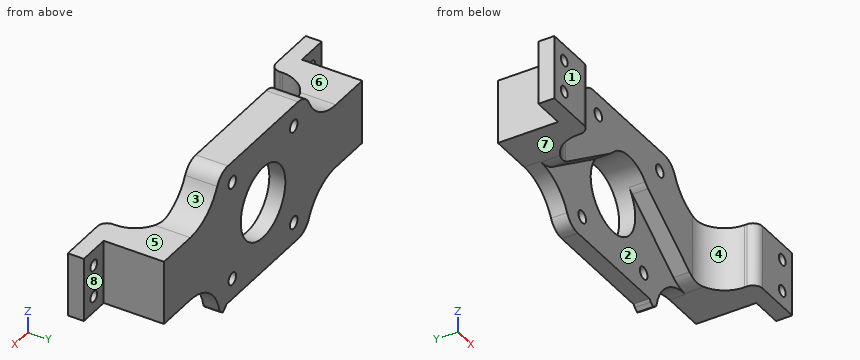
```python
from build123d import *

# Parameters (mm, degrees)
AUFSATZ_LINEAR_AUSTRAGEN1_DEPTH      = 10
SKIZZE6_R                            = 1.9
SKIZZE6_R_2                          = 11.25
SCHNITT_LINEAR_AUSTRAGEN4_DEPTH      = 67.632124385
SKIZZE7_W                            = 20.880821379
SKIZZE7_H                            = 5
SCHNITT_LINEAR_AUSTRAGEN5_DEPTH      = 87.970339772
VERRUNDUNG3_R                        = 15
SCHNITT_LINEAR_AUSTRAGEN6_DEPTH      = 69.73136111
SCHNITT_LINEAR_AUSTRAGEN6_DEPTH_BACK = 69.73136111
SKIZZE8_W                            = 10
SKIZZE8_H                            = 10
AUFSATZ_LINEAR_AUSTRAGEN4_DEPTH      = 20
VERRUNDUNG7_R                        = 10
VERRUNDUNG8_R                        = 3
SKIZZE16_R                           = 1.7
SCHNITT_LINEAR_AUSTRAGEN8_DEPTH      = 10
AUFSATZ_LINEAR_AUSTRAGEN6_DEPTH      = 5
VERRUNDUNG9_R                        = 0.5
FASE1_START                          = -13.795598923
FASE1_DEPTH                          = 18.795598923
VERRUNDUNG10_R                       = 10
VERRUNDUNG11_R                       = 6


with BuildPart() as part:
    # Skizze1 → Aufsatz-Linear austragen1 (new body)
    with BuildSketch(Plane(origin=(0, 0, 0), x_dir=(1, 0, 0), z_dir=(0, 1, 0))):
        Polygon((-60, -4.8), (-22, -4.8), (-22, -16.8), (22, -16.8), (22, -4.8), (60, -4.8), (60, 15.2), (22, 15.2), (22, 27.2), (0, 27.2), (-22, 27.2), (-22, 15.2), (-60, 15.2), align=None)
    extrude(amount=AUFSATZ_LINEAR_AUSTRAGEN1_DEPTH)

    # Skizze6 → Schnitt-Linear austragen4 (cut, through all)
    with BuildSketch(Plane(origin=(0, 10, 0), x_dir=(1, 0, 0), z_dir=(0, 1, 0))):
        with Locations(Location((15.5, 20.7, 0), (0, 0, 270))):
            Circle(SKIZZE6_R)
        with Locations(Location((15.5, -10.3, 0), (0, 0, 270))):
            Circle(SKIZZE6_R)
        with Locations(Location((-15.5, -10.3, 0), (0, 0, 270))):
            Circle(SKIZZE6_R)
        with Locations(Location((-15.5, 20.7, 0), (0, 0, 270))):
            Circle(SKIZZE6_R)
        with Locations(Location((0, 5.2, 0), (0, 0, 270))):
            Circle(SKIZZE6_R_2)
    extrude(amount=-SCHNITT_LINEAR_AUSTRAGEN4_DEPTH, mode=Mode.SUBTRACT)

    # Skizze7 → Schnitt-Linear austragen5 (cut, through all)
    with BuildSketch(Plane.ZY.offset(22)):
        with Locations((-25.64041069, 2.5)):
            Rectangle(SKIZZE7_W, SKIZZE7_H)
    extrude(amount=-SCHNITT_LINEAR_AUSTRAGEN5_DEPTH, mode=Mode.SUBTRACT)

    # Verrundung3
    # the kernel refuses this fillet: 15 mm, written as the material it adds along each edge
    with BuildSketch(Plane(origin=(-22, 5, -15.2), x_dir=(0, 0, -1), z_dir=(0, 1, 0))) as verrundung3_piece_1:
        with BuildLine():
            CenterArc((15, 14.696938457), VERRUNDUNG3_R, 180, 78.463040967)
            Line((0, 14.696938457), (-0.3, 14.696938457))
            Line((-0.3, 14.696938457), (-0.3, 0))
            Line((-0.3, 0), (0, -0.3))
            ThreePointArc((0, -0.3), (6, -0.3), (11.94, -0.293938769))
            Line((11.94, -0.293938769), (12, 0))
        make_face()
    extrude(amount=5)
    with BuildSketch(Plane(origin=(-22, 0, 4.8), x_dir=(-1, 0, 0), z_dir=(0, 1, 0))) as verrundung3_piece_2:
        with BuildLine():
            CenterArc((14.696938457, 15), VERRUNDUNG3_R, 191.536959033, 78.463040967)
            Line((0, 12), (-0.293938769, 11.94))
            ThreePointArc((-0.293938769, 11.94), (-0.3, 6), (-0.3, 0))
            Line((-0.3, 0), (0, -0.3))
            Line((0, -0.3), (14.696938457, -0.3))
            Line((14.696938457, -0.3), (14.696938457, 0))
        make_face()
    extrude(amount=10)
    with BuildSketch(Plane(origin=(22, 0, 4.8), x_dir=(1, 0, 0), z_dir=(0, 1, 0))) as verrundung3_piece_3:
        with BuildLine():
            CenterArc((14.696938457, -15), VERRUNDUNG3_R, 90, 78.463040967)
            Line((0, -12), (-0.293938769, -11.94))
            ThreePointArc((-0.293938769, -11.94), (-0.3, -6), (-0.3, 0))
            Line((-0.3, 0), (0, 0.3))
            Line((0, 0.3), (14.696938457, 0.3))
            Line((14.696938457, 0.3), (14.696938457, 0))
        make_face()
    extrude(amount=10)
    with BuildSketch(Plane(origin=(22, 5, -15.2), x_dir=(1, 0, 0), z_dir=(0, 1, 0))) as verrundung3_piece_4:
        with BuildLine():
            CenterArc((14.696938457, 15), VERRUNDUNG3_R, 191.536959033, 78.463040967)
            Line((0, 12), (-0.293938769, 11.94))
            ThreePointArc((-0.293938769, 11.94), (-0.3, 6), (-0.3, 0))
            Line((-0.3, 0), (0, -0.3))
            Line((0, -0.3), (14.696938457, -0.3))
            Line((14.696938457, -0.3), (14.696938457, 0))
        make_face()
    extrude(amount=5)

    # Skizze8 → Schnitt-Linear austragen6 (cut, two sides: drawn at the far end of the back side and taken through both)
    with BuildSketch(Plane(origin=(0, 0, -15.2), x_dir=(-1, 0, 0), z_dir=(0, 0, -1)).offset(-SCHNITT_LINEAR_AUSTRAGEN6_DEPTH_BACK)):
        with Locations((-55, 5)):
            Rectangle(SKIZZE8_W, SKIZZE8_H)
        with Locations((55, 5)):
            Rectangle(SKIZZE8_W, SKIZZE8_H)
    extrude(amount=SCHNITT_LINEAR_AUSTRAGEN6_DEPTH + SCHNITT_LINEAR_AUSTRAGEN6_DEPTH_BACK, mode=Mode.SUBTRACT)

    # Skizze12 → Aufsatz-Linear austragen4 (add)
    with BuildSketch(Plane(origin=(0, 0, -15.2), x_dir=(-1, 0, 0), z_dir=(0, 0, -1))):
        Polygon((-50, 0), (-50, -8.795598923), (-60, -8.795598923), (-60, -13.795598923), (-42.093723734, -13.795598923), (-42.093723734, 0), align=None)
        Polygon((50, 0), (42.093723734, 0), (42.093723734, -13.795598923), (60, -13.795598923), (60, -8.795598923), (50, -8.795598923), align=None)
    extrude(amount=-AUFSATZ_LINEAR_AUSTRAGEN4_DEPTH)

    # Verrundung7
    verrundung7_edges = [part.edges().sort_by_distance(p)[0] for p in [
        (42.093723734, 0, -5.2),
        (-42.093723734, 0, -5.2),
    ]]
    fillet(verrundung7_edges, radius=VERRUNDUNG7_R)

    # Verrundung8
    verrundung8_edges = [part.edges().sort_by_distance(p)[0] for p in [
        (42.093723734, -13.795598923, -5.2),
        (-42.093723734, -13.795598923, -5.2),
    ]]
    fillet(verrundung8_edges, radius=VERRUNDUNG8_R)

    # Skizze16 → Schnitt-Linear austragen8 (cut)
    with BuildSketch(Plane.XZ.offset(13.795598923)):
        with Locations(Location((-55, -10.2, 0), (0, 0, 270))):
            Circle(SKIZZE16_R)
        with Locations(Location((-55, -0.2, 0), (0, 0, 180))):
            Circle(SKIZZE16_R)
        with Locations(Location((55, -0.2, 0), (0, 0, 270))):
            Circle(SKIZZE16_R)
        with Locations(Location((55, -10.2, 0), (0, 0, 180))):
            Circle(SKIZZE16_R)
    extrude(amount=-SCHNITT_LINEAR_AUSTRAGEN8_DEPTH, mode=Mode.SUBTRACT)

    # Skizze17 → Aufsatz-Linear austragen6 (add)
    with BuildSketch(Plane.XZ.offset(-5)):
        Polygon((22, -27.2), (20.323301152, -27.2), (20.323301152, -28.736029672), (21.681082582, -27.841522035), align=None)
        Polygon((20.323301152, -28.736029672), (20.323301152, -27.2), (18.646602303, -27.2), (18.965519721, -27.841522035), align=None)
    extrude(amount=-AUFSATZ_LINEAR_AUSTRAGEN6_DEPTH)

    # Verrundung9
    verrundung9_edges = [part.edges().sort_by_distance(p)[0] for p in [
        (22, 7.5, -27.2),
        (18.646602303, 7.5, -27.2),
        (21.681082582, 7.5, -27.841522035),
        (18.965519721, 7.5, -27.841522035),
    ]]
    fillet(verrundung9_edges, radius=VERRUNDUNG9_R)

    # Fase1: read off the stored shape, not the designer's step
    # Fase1 outline → Fase1 (cut)
    with BuildSketch(Plane(origin=(0, 0, 0), x_dir=(1, 0, 0), z_dir=(0, 1, 0)).offset(FASE1_START)):
        with BuildLine():
            Line((-5.153882032, 15.2), (-33.153882032, 15.2))
            Line((-33.153882032, 15.2), (-8.71856035, -1.90979644))
            ThreePointArc((-8.71856035, -1.90979644), (-11.013512063, 7.494570119), (-5.153882032, 15.2))
        make_face()
        with BuildLine():
            ThreePointArc((5.153882032, 15.2), (11.013512063, 7.494570119), (8.71856035, -1.90979644))
            Line((8.71856035, -1.90979644), (33.153882032, 15.2))
            Line((33.153882032, 15.2), (5.153882032, 15.2))
        make_face()
    extrude(amount=FASE1_DEPTH, mode=Mode.SUBTRACT)

    # Verrundung10
    verrundung10_edges = [part.edges().sort_by_distance(p)[0] for p in [
        (-8.71856035, 2.5, 1.90979644),
        (8.71856035, 2.5, 1.90979644),
        (-33.153882032, 2.471822211, -15.2),
        (33.153882032, 2.471822211, -15.2),
    ]]
    fillet(verrundung10_edges, radius=VERRUNDUNG10_R)

    # Verrundung11
    verrundung11_edges = [part.edges().sort_by_distance(p)[0] for p in [
        (22, 5, 16.8),
        (-22, 5, 16.8),
        (-22, 7.5, -27.2),
    ]]
    fillet(verrundung11_edges, radius=VERRUNDUNG11_R)


solid = part.part
```
Geometry check sheet. Reference: the model listing, model coordinates, mm. Face numbers are marked on the shaded views. A direction names the side the tool comes from. Give positions to 0.01 mm unless a question says otherwise; leave off trailing zeros. Write each loop counter-clockwise with the first axis right and the second up, starting at its lowest first coordinate (ties: lowest second). Pieces come first, ordered by that corner, then holes. Notation, with made-up numbers: (-33, -34) -> (-11, -34) arc R17 cw to (-11, -29) -> close; hole circle Ø9 at (-4, 28). An arc over 180 degrees is marked (long way). One line per question, with ' | ' between items.
Item 1: Draft check along X on the marked faces 1, 2 and 3. Enter one of: released by +X, released by -X, zero draft, split by the parting line, or undercut.
Determined:
face 1: zero draft | face 2: undercut | face 3: released by +X
Item 2: Depth check by flat-ended pin: pin 1 (2.5 mm diameter, centred on x = 15.5, z = -20.7, fed in from +Y); pin 2 (8 mm diameter, centred on x = -56, z = -4, fed in from +Y); pin 3 (9.5 mm diameter, centred on y = 0.5, z = -4.5, fed in from +X); pin 4 (1.5 mm diameter, centred on x = 42, y = -3.5, fed in from +Z). Enter the tip coordinate at first touch or a pass-through.
Determined:
pin 1: through | pin 2: y = -8.8 | pin 3: x = 50 | pin 4: z = 4.8
Item 3: Sectioned sample at C-C, the plane z = -0.2. State how many separate pieces and enclosed holes the cut face has, plus the area to 3 significant figures.
Determined:
separate pieces: 4 | enclosed holes: 0 | area: 1,110 mm^2
Item 4: Sectioned sample at D-D, the plane y = -7.75. Record the boundary of the cut face in (x, z), plus the area to 3 significant figures.
Determined:
outline: (-50, -15.2) -> (-41.84, -15.2) -> (-41.84, 4.8) -> (-50, 4.8) -> close; (41.84, -15.2) -> (50, -15.2) -> (50, 4.8) -> (41.84, 4.8) -> close | area: 327 mm^2
Item 5: Access from +Z, -Z, +X, -X, +Y, -Y to the whole of each face (thin tool, end or side, straight path). Record for the marked faces 4, 5, 6, 7 and 8.
Determined:
face 4: +Z, -Z, -Y | face 5: +Z, +X, +Y, -Y | face 6: +Z, -X, +Y, -Y | face 7: -Z, -X, +Y, -Y | face 8: +Z, -Z, +X, +Y
Item 6: Sectioned sample at A-A, the plane x = 55. Record the boundary of the cut face in (y, z), plus the area to 3 significant figures.
Determined:
outline: (-13.8, -15.2) -> (-8.8, -15.2) -> (-8.8, -11.9) -> (-13.8, -11.9) -> close; (-13.8, -8.5) -> (-8.8, -8.5) -> (-8.8, -1.9) -> (-13.8, -1.9) -> close; (-13.8, 1.5) -> (-8.8, 1.5) -> (-8.8, 4.8) -> (-13.8, 4.8) -> close | area: 66.0 mm^2
Item 7: Sectioned sample at B-B, the plane x = 0. Record the boundary of the cut face in (y, z).
Determined:
outline: (0, 6.05) -> (10, 6.05) -> (10, 16.8) -> (0, 16.8) -> close; (5, -27.2) -> (10, -27.2) -> (10, -16.45) -> (5, -16.45) -> close
Item 8: Scan lines: line 1 along X through (y, z) = (-11.05, -10.2); line 2 along Z through (x, y) = (0, 6.75); line 3 along X through (y, z) = (7.5, -5.2). Record each from-to range of solid material in increasing order.
Determined:
line 1: -60 to -56.7, -53.3 to -42.1, 42.1 to 53.3, 56.7 to 60 | line 2: -27.2 to -16.45, 6.05 to 16.8 | line 3: -50 to -11.25, 11.25 to 50
